Solid Edge part; units mm, degrees
sketch "Sketch1" plane through (0, 0, 0) normal (0, 0, 1) x (1, 0, 0)
  line L0 (-6.1009, 4.0673) -> (-6.5728, -3.2499)
  line L1 (-6.5728, -3.2499) -> (-0.4719, -7.3171)
  line L2 (-0.4719, -7.3171) -> (6.1009, -4.0673)
  line L3 (6.1009, -4.0673) -> (6.5728, 3.2499)
  line L4 (6.5728, 3.2499) -> (0.4719, 7.3171)
  line L5 (0.4719, 7.3171) -> (-6.1009, 4.0673)
extrude "Protrusion1" add sketch "Sketch1" against normal blind 80
sketch "Sketch2" plane through (0, 0, -2) normal (0, 0, 1) x (-0.8964, -0.4432, 0)
  circle A0 centre (0, 0) radius 5.5
  circle A1 centre (0, 0) radius 13.1424
extrude "ExtrudedCutout_1" cut sketch "Sketch2" against normal blind 2
sketch "Sketch3" plane through (0, 0, -78) normal (0, 0, -1) x (0.8964, 0.4432, 0)
  circle A0 centre (0, 0) radius 5.5
  circle A1 centre (0, 0) radius 13.1424
extrude "ExtrudedCutout_2" cut sketch "Sketch3" against normal blind 2
properties part number "BumbleB0196"
Read the model definition and answer for the solid it produces. Units are mm, in the model's axes. A direction names the side the tool comes from. Round coordinates to 2 decimals unless told otherwise and drop trailing zeros. Write each loop counter-clockwise with the first axis right and the second up, starting at its lowest first coordinate (ties: lowest second). Pieces come first, ordered by that corner, then holes. Notation, with made-up numbers: (-5, 65) -> (54, 65) arc R35 cw to (54, 100) -> close; hole circle Ø9 at (-39, 67.25). An arc over 180 degrees is marked (long way). Answer in a Markdown table with one row per item. Add a question column.
1) Consider line 1 (Z direction, x = -4.5, y = 3.75); line 2 (X direction, y = 3.25, z = -47); line 3 (X direction, y = 4.5, z = -24). Determine where each line is inside the solid, lowest interval first.
2) Given P1, Ø1.5, axis at y = 4.5, z = -69.5, coming from the +X side; P2, Ø3, axis at x = 4.5, z = -20.5, coming from the -Y side, each flat-ended and moving along its own axis, determine where each tip first touches the part or whether it passes through.
3) Determine the mould class of faces 1 (the face through (6.334, -0.46, -39.496)), 2 (the face through (0, 0, 0)), 3 (the face through (0, 0, -80)), 4 (the face through (5, -3, -78)) for opening direction Z: pulls with the +Z half, pulls with the -Z half, needs draft (parallel to the pull), parting line crosses it, or undercut.
4) Find section A-A, the plane z = -41.5. Determine the outline of the cut face in (x, y).
5) Find section B-B, the plane y = 0. Determine the outline of the cut face in (x, z), and give its area (3 significant figures).
6) Which of the six approach directions +Z, -Z, +X, -X, +Y, -Y give full straight-line access (tool end or side, diameter ignored) to faces 5 (the face through (-5, -3, -4)), 6 (the face through (3.565, 5.255, -0.986))?
7) Find section C-C, the plane x = -3.25. Determine the outline of the cut face in (y, z), and give its area (3 significant figures).
Findings below:
| question | item | result |
|---|---|---|
| 1 | line 1 | -80 to -78, -76 to -4, -2 to 0 |
| 1 | line 2 | -6.15 to 6.57 |
| 1 | line 3 | -5.23 to 4.7 |
| 2 | P1 | x = 5.82 |
| 2 | P2 | y = -5.6 |
| 3 | face 1 | needs draft |
| 3 | face 2 | pulls with the +Z half |
| 3 | face 3 | pulls with the -Z half |
| 3 | face 4 | undercut |
| 4 | outline | (-6.57, -3.25) -> (-0.47, -7.32) -> (6.1, -4.07) -> (6.57, 3.25) -> (0.47, 7.32) -> (-6.1, 4.07) -> close |
| 5 | outline | (-6.36, -80) -> (6.36, -80) -> (6.36, -78) -> (5.5, -78) -> (5.5, -76) -> (6.36, -76) -> (6.36, -4) -> (5.5, -4) -> (5.5, -2) -> (6.36, -2) -> (6.36, 0) -> (-6.36, 0) -> (-6.36, -2) -> (-5.5, -2) -> (-5.5, -4) -> (-6.36, -4) -> (-6.36, -76) -> (-5.5, -76) -> (-5.5, -78) -> (-6.36, -78) -> close |
| 5 | area | 1,010 mm² |
| 6 | face 5 | none |
| 6 | face 6 | +Z, -Z, +X, +Y |
| 7 | outline | (-5.47, -80) -> (5.48, -80) -> (5.48, -78) -> (4.44, -78) -> (4.44, -76) -> (5.48, -76) -> (5.48, -4) -> (4.44, -4) -> (4.44, -2) -> (5.48, -2) -> (5.48, 0) -> (-5.47, 0) -> (-5.47, -2) -> (-4.44, -2) -> (-4.44, -4) -> (-5.47, -4) -> (-5.47, -76) -> (-4.44, -76) -> (-4.44, -78) -> (-5.47, -78) -> close |
| 7 | area | 867 mm² |
